Work out the finished part from the listing and answer in its coordinate system (mm). A direction names the side the tool comes from. Round coordinates to 2 decimals unless told otherwise and drop trailing zeros. Order: outer loops, then holes, each group sorted by start corner. A loop starts at its lowest first (then second) coordinate and runs counter-clockwise, first axis right, second up. Notation, with made-up numbers: (16.5, 3) - (68.5, 3) arc R19 ccw to (68.5, 30) - close; hole circle Ø9 at (34, -28.75). An arc over 180 degrees is marked (long way). Use one line per item in the form item = value. Start each with the question number.
Q1. Which of the six approach directions +Z, -Z, +X, -X, +Y, -Y give full straight-line access (tool end or side, diameter ignored) to faces 4 (the flat face through (0, 85, 2)), 5 (the flat face through (0, 84.5, 2))?
Q2. The part is cut by section A-A on x = 0. Determine the outline of the cut face in (y, z) (3 decimals), plus the area to 3 significant figures.
Q3. The part is cut by section B-B on z = 2.45. Determine the outline of the cut face in (x, y) (3 decimals).
Q4. For a pull along X with two mould halves and no side action, classify faces 1 (the flat face through (6, -1, 2)), 2 (the flat face through (0, 1, 0)), 3 (the flat face through (0, 84.2, 3.5)) as +X half, -X half, draft (parallel to the pull), parting line (faces both ways), or undercut.
Q5. Find the intervals of material crossed by line 1 (X direction, y = -65, z = 1.4); line 2 (Y direction, x = 0.75, z = 1.65); line 3 (Y direction, x = -4, z = 2.6), in increasing order. Write a range as [from, to].
from build123d import *

# Parameters (mm, degrees)
SKETCH_W     = 12
SKETCH_H     = 170
SKETCH_W_2   = 6.05
SKETCH_H_2   = 6.05
PAD_DEPTH    = 4
SKETCH001_W  = 6.05
SKETCH001_H  = 6.05
PAD001_DEPTH = 0.5
SKETCH002_R  = 2.5
POCKET_DEPTH = 0.5
SKETCH003_R  = 1.2
HOLE_DEPTH   = 25


with BuildPart() as part:
    # Sketch → Pad (new body)
    with BuildSketch(Plane.XY):
        Rectangle(SKETCH_W, SKETCH_H)
        with Locations((0, 81.475)):
            Rectangle(SKETCH_W_2, SKETCH_H_2, mode=Mode.SUBTRACT)
    extrude(amount=PAD_DEPTH)

    # Sketch001 (on Face10 of Pad) → Pad001 (join)
    with BuildSketch(Plane.XY.offset(4)):
        with Locations((0, 81.475)):
            Rectangle(SKETCH001_W, SKETCH001_H)
    extrude(amount=-PAD001_DEPTH)

    # Sketch002 (on Face11 of Pad001) → Pocket (cut)
    with BuildSketch(Plane.XY.offset(4)):
        with Locations((0, 81.475)):
            Circle(SKETCH002_R)
    extrude(amount=-POCKET_DEPTH, mode=Mode.SUBTRACT)

    # Sketch003 (on Face5 of Pocket) → Hole (cut)
    with BuildSketch(Plane.XY.offset(4)):
        with Locations((3, 58.45)):
            Circle(SKETCH003_R)
        with Locations((-3, 58.45)):
            Circle(SKETCH003_R)
        with Locations((3, -3.275)):
            Circle(SKETCH003_R)
        with Locations((-3, -3.275)):
            Circle(SKETCH003_R)
        with Locations((3, -65)):
            Circle(SKETCH003_R)
        with Locations((-3, -65)):
            Circle(SKETCH003_R)
    extrude(amount=-HOLE_DEPTH, mode=Mode.SUBTRACT)


solid = part.part
Found:
q1.face_4 = +Z, -Z, +X, -X, +Y
q1.face_5 = -Z
q2.outline = (-85, 0) - (78.45, 0) - (78.45, 3.5) - (78.975, 3.5) - (78.975, 4) - (-85, 4) - close; (83.975, 3.5) - (84.5, 3.5) - (84.5, 0) - (85, 0) - (85, 4) - (83.975, 4) - close
q2.area = 656 mm²
q3.outline = (-6, -85) - (6, -85) - (6, 85) - (-6, 85) - close; hole circle Ø2.4 at (-3, -65); hole circle Ø2.4 at (-3, -3.275); hole circle Ø2.4 at (-3, 58.45); hole (-3.025, 78.45) - (3.025, 78.45) - (3.025, 84.5) - (-3.025, 84.5) - close; hole circle Ø2.4 at (3, -65); hole circle Ø2.4 at (3, -3.275); hole circle Ø2.4 at (3, 58.45)
q4.face_1 = +X half
q4.face_2 = draft
q4.face_3 = undercut
q5.line_1 = [-6, -4.2], [-1.8, 1.8], [4.2, 6]
q5.line_2 = [-85, 78.45], [84.5, 85]
q5.line_3 = [-85, -65.66], [-64.34, -3.94], [-2.61, 57.79], [59.11, 85]
